Can you work these out from the drawing? Everything is in mm from the part's minimum corner. A direction names the side the tool comes from. Coordinates: 2 decimals unless noted, no trailing zeros. Loops run counter-clockwise (first coordinate to the right, second up) from the corner with the lowest first, then second, coordinate; pieces in that order, holes last. Notation, with made-up numbers: (81, 78) -> (125, 78) arc R26 cw to (125, 112) -> close; hole circle Ø7 at (9, -38.75). An arc over 180 degrees is marked (long way). Put each result on its own line as item: value. Start each with the question number.
Item 1: If we section it at C-C on x = 4: Please give me the cut outline in (y, z), plus the area to 3 significant figures.
Item 2: If we section it at B-B on y = 3.35: Please give me the cut outline in (x, z) (3 decimals).
Item 3: Will this pin go through, and if not, where does the flat tip stop? P1, Ø4.5, axis at x = 37.842, z = 37.842, coming from the +Y side.
Item 4: If we section it at D-D on z = 33: Please give me the cut outline in (x, y), plus the area to 3 significant figures.
Item 5: We'd pull the mould along X, two halves only. Please class the marked faces 3, 4 and 5: pulls with the +X half, pulls with the -X half, needs draft (parallel to the pull), parting line crosses it, or undercut.
Item 6: If we section it at A-A on z = 11: Please give me the cut outline in (x, y).
Item 7: For the marked faces 1 and 2, which set-ups out of +Z, -Z, +X, -X, +Y, -Y let a thin tool reach every point of the face, with its end or its side?
Item 8: Please list where these lines run through material, in increasing order: L1, parallel to X at y = 1.4, z = 37; L2, parallel to Z at x = 38.5, y = 4.4. Write a range as from..to.
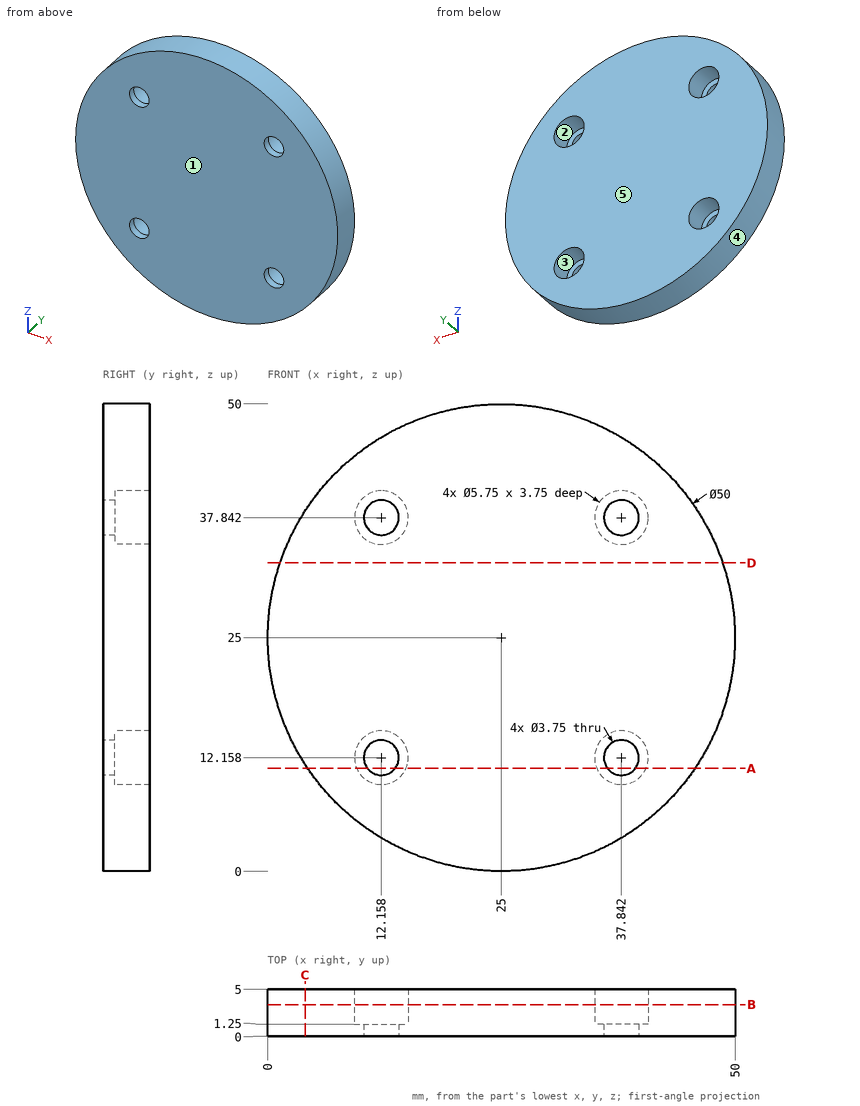
Solutions:
1. outline: (0, 11.44) -> (5, 11.44) -> (5, 38.56) -> (0, 38.56) -> close
1. area: 136 mm^2
2. outline: circle Ø50 at (25, 25); hole circle Ø5.75 at (12.158, 12.158); hole circle Ø5.75 at (12.158, 37.842); hole circle Ø5.75 at (37.842, 12.158); hole circle Ø5.75 at (37.842, 37.842)
3. P1: y = 1.25
4. outline: (1.31, 0) -> (48.69, 0) -> (48.69, 5) -> (1.31, 5) -> close
4. area: 237 mm^2
5. face 3: undercut
5. face 4: parting line crosses it
5. face 5: needs draft
6. outline: (4.29, 0) -> (10.68, 0) -> (10.68, 1.25) -> (9.53, 1.25) -> (9.53, 5) -> (4.29, 5) -> close; (13.63, 0) -> (36.37, 0) -> (36.37, 1.25) -> (35.21, 1.25) -> (35.21, 5) -> (14.79, 5) -> (14.79, 1.25) -> (13.63, 1.25) -> close; (39.32, 0) -> (45.71, 0) -> (45.71, 5) -> (40.47, 5) -> (40.47, 1.25) -> (39.32, 1.25) -> close
7. face 1: +Z, -Z, +X, -X, -Y
7. face 2: +Y
8. L1: 3.07..9.41, 14.91..35.09, 40.59..46.93
8. L2: 3.96..9.36, 14.96..35.04, 40.64..46.04
